Source: CAD feature listing. Evaluate the final solid. Frame: model axes, mm. Face numbers are marked on the shaded views. A direction names the side the tool comes from. Round coordinates to 2 decimals unless told otherwise and drop trailing zeros. Order: outer loops, then holes, each group sorted by start corner. A loop starts at its lowest first (then second) coordinate and runs counter-clockwise, first axis right, second up. Notation, with made-up numbers: M -11.5,70 L 0.5,70 A17 ccw 0.5,94 Z; hole C 75.5,-12 d5. An arc over 180 degrees is marked long. Answer in a Markdown table with one row per item. Add a question column.
Autodesk Inventor part; units mm, degrees
ref_plane "YZ Plane" through (0, 0, 0) normal (1, 0, 0) x (0, 1, 0)
ref_plane "XZ Plane" through (0, 0, 0) normal (0, 1, 0) x (-1, 0, 0)
ref_plane "XY Plane" through (0, 0, 0) normal (0, 0, 1) x (1, 0, 0)
sketch "スケッチ1" plane through (0, 0, 0) normal (0, 0, 1) x (1, 0, 0)
  circle A0 centre (0, 0) radius 21
  dimension "d0" = 42
extrude "押し出し1" add sketch "スケッチ1" along normal blind 32
sketch "スケッチ2" plane through (0, 0, 32) normal (0, 0, 1) x (1, 0, 0)
  circle A0 centre (0, 0) radius 12.5
  dimension "d3" = 25
extrude "押し出し2" add sketch "スケッチ2" along normal blind 2
sketch "スケッチ3" plane through (0, 0, 34) normal (0, 0, 1) x (1, 0, 0)
  circle A0 centre (0, 0) radius 4
  dimension "d6" = 8
extrude "押し出し3" add sketch "スケッチ3" along normal blind 20
sketch "スケッチ4" plane through (0, 0, 32) normal (0, 0, 1) x (1, 0, 0)
  point P0 (0, 0)
  point P1 (0, 17.5)
  point P2 (-17.5, 0)
  point P3 (0, -17.5)
  point P4 (17.5, 0)
  dimension "d9" = 17.5
  dimension "d12" = 360
hole "穴1" at (0, 17.5, 32) at (-17.5, 0, 32) at (0, -17.5, 32) at (17.5, 0, 32) direction (0, 0, -1) diameter 4 depth 8 tip angle 118
properties part number "775_gearhead" material "鉄、ねずみ鋳鉄"
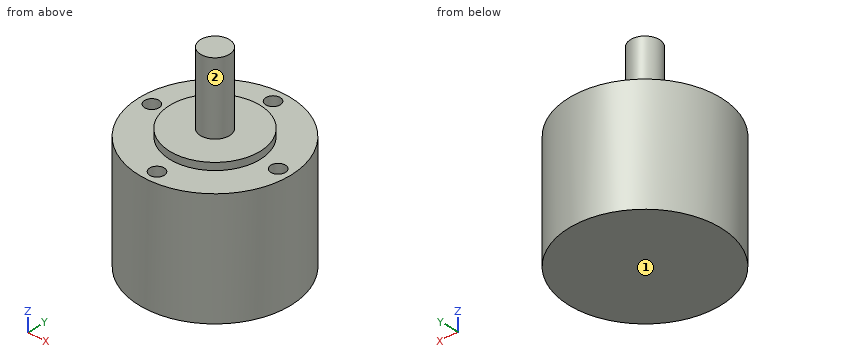
(1) Line query: line 1 (Y direction, x = 0, z = 27); line 2 (Z direction, x = -8, y = 7.5); line 3 (Z direction, x = -6.5, y = 14). Output: solid intervals per line, ascending. Write a range as from..to.
(2) Cut plane D-D (z = 41). Return loops of the section in (x, y), and give its area (3 significant figures).
(3) Access query for the marked faces 1 and 2. Directions: +Z, -Z, +X, -X, +Y, -Y. A direction counts if a zero-diameter tool reaches every point of the face in a straight line with its end or side. Return the directions, or none.
(4) Cut plane A-A (x = -7). Return loops of the section in (y, z).
(5) Pin query (flat end, axial travel): pin 1 (10 mm diameter, centred on y = -12.5, z = 35, fed in from -X); pin 2 (2 mm diameter, centred on x = 6, z = 37.5, fed in from +Y); pin 3 (3 mm diameter, centred on y = -8, z = 8, fed in from -X); pin 4 (3 mm diameter, centred on x = 0, y = -17.5, fed in from +Z). Return the tip coordinate at first contact, or that it passes through.
(6) Cut plane C-C (y = 5.5). Return loops of the section in (x, z).
(7) Cut plane B-B (z = 9.5). Return loops of the section in (x, y), and give its area (3 significant figures).
Answer list:
| question | item | result |
|---|---|---|
| 1 | line 1 | -21..-19.5, -15.5..15.5, 19.5..21 |
| 1 | line 2 | 0..34 |
| 1 | line 3 | 0..32 |
| 2 | outline | C 0,0 d8 |
| 2 | area | 50.3 mm² |
| 3 | face 1 | -Z, +X, -X, +Y, -Y |
| 3 | face 2 | +Z |
| 4 | outline | M -19.8,0 L 19.8,0 L 19.8,32 L 10.36,32 L 10.36,34 L -10.36,34 L -10.36,32 L -19.8,32 Z |
| 5 | pin 1 | x = -19.2 |
| 5 | pin 2 | through |
| 5 | pin 3 | x = -19.97 |
| 5 | pin 4 | z = 23.7 |
| 6 | outline | M -20.27,0 L 20.27,0 L 20.27,32 L 11.22,32 L 11.22,34 L -11.22,34 L -11.22,32 L -20.27,32 Z |
| 7 | outline | C 0,0 d42 |
| 7 | area | 1,390 mm² |
